Read the model definition and answer for the solid it produces. Units are mm, in the model's axes. A direction names the side the tool comes from. Give positions to 0.01 mm unless a question says otherwise; leave off trailing zeros. Write each loop counter-clockwise with the first axis right and the second up, starting at its lowest first coordinate (ties: lowest second). Pieces come first, ordered by that corner, then holes. Notation, with made-up numbers: (3, 87.25) -> (54, 87.25) arc R18 ccw to (54, 122.25) -> close; hole circle Ø6 at (12, 19.25). An arc over 180 degrees is marked (long way). Use a Markdown table: item, result.
from build123d import *

# Parameters (mm, degrees)
CHANFREIN2_SIZE  = 0.6
CHANFREIN2_SIZE2 = 0.218382141
CHANFREIN3_SIZE  = 0.3
CHANFREIN4_SIZE  = 0.2
CONG_1_R         = 0.4


with BuildPart() as part:
    # Esquisse1 → Base-Révolution (revolve)
    with BuildSketch(Plane.XY, mode=Mode.PRIVATE) as base_r_volution_sk:
        Polygon((-1, 6), (-1, 10), (0, 10), (0, 7), (8, 7), (8, 6), align=None)
    revolve(base_r_volution_sk.sketch.rotate(Axis((-5.312682662, 0, 0), (1, 0, 0)), 90), axis=Axis((-5.312682662, 0, 0), (1, 0, 0)))

    # Chanfrein2
    chanfrein2_edges = [part.edges().sort_by_distance(p)[0] for p in [
        (8, 0, -7),
    ]]
    chanfrein2_side = [part.faces().sort_by_distance(p)[0] for p in [
        (4, 0, -7),
    ]]
    chamfer(chanfrein2_edges, length=CHANFREIN2_SIZE, length2=CHANFREIN2_SIZE2, reference=chanfrein2_side[0])

    # Chanfrein3
    chanfrein3_edges = [part.edges().sort_by_distance(p)[0] for p in [
        (-1, 0, -6),
        (8, 0, -6),
    ]]
    chamfer(chanfrein3_edges, length=CHANFREIN3_SIZE)

    # Chanfrein4
    chanfrein4_edges = [part.edges().sort_by_distance(p)[0] for p in [
        (0, 0, -10),
        (-1, 0, -10),
    ]]
    chamfer(chanfrein4_edges, length=CHANFREIN4_SIZE)

    # Congé1
    cong_1_edges = [part.edges().sort_by_distance(p)[0] for p in [
        (0, 0, -7),
    ]]
    fillet(cong_1_edges, radius=CONG_1_R)


solid = part.part
Item 1: A cutting plane is placed at A-A (z = 0). Give the vertices of the cut face in (x, y), then the cut area to 3 significant figures.
Return value:
| item | result |
|---|---|
| outline | (-1, -9.8) -> (-0.8, -10) -> (-0.2, -10) -> (0, -9.8) -> (0, -7.4) arc R0.4 cw to (0.4, -7) -> (7.4, -7) -> (8, -6.78) -> (8, -6.3) -> (7.7, -6) -> (-0.7, -6) -> (-1, -6.3) -> close; (-1, 6.3) -> (-0.7, 6) -> (7.7, 6) -> (8, 6.3) -> (8, 6.78) -> (7.4, 7) -> (0.4, 7) arc R0.4 cw to (0, 7.4) -> (0, 9.8) -> (-0.2, 10) -> (-0.8, 10) -> (-1, 9.8) -> close |
| area | 23.7 mm^2 |
Item 2: Straight lines are drawn through the part: line 1 along Y through (x, z) = (1.25, 0); line 2 along Z through (x, y) = (5.75, 0.25); line 3 along X through (y, z) = (-6.75, 6.25). For each, find the intervals that lie inside material, in ascending order. Write a range as [from, to].
Return value:
| item | result |
|---|---|
| line 1 | [-7, -6], [6, 7] |
| line 2 | [-7, -5.99], [5.99, 7] |
| line 3 | [-1, 0] |
Item 3: A tool of negligible diameter and unlimited length cuts with its end or side. For faces 4 (the face through (3.95, 6.21, 3.23)), 5 (the face through (-1, 6.4, -2)), from which of +Z, -Z, +X, -X, +Y, -Y can it reach the whole face along a straight path? Write none if from no direction.
Return value:
| item | result |
|---|---|
| face 4 | +X |
| face 5 | +Z, -Z, -X, +Y, -Y |
Item 4: Each of these flat-tipped pins is pushed along its axis until it touches: P1, Ø5, axis at x = 7, z = -7.5, coming from the +Y side; P2, Ø4, axis at x = 6, z = 4, coming from the +Y side; P3, Ø5, axis at x = 1, y = -7, coming from the -Z side. Where does it stop, or does it pass through?
Return value:
| item | result |
|---|---|
| P1 | y = 4.9 |
| P2 | y = 6.71 |
| P3 | z = -8.77 |
Item 5: A cutting plane is placed at C-C (x = 3.75). Give the vertices of the cut face in (y, z).
Return value:
| item | result |
|---|---|
| outline | circle Ø14 at (0, 0); hole circle Ø12 at (0, 0) |
Item 6: For a pull along Z with two mould halves and no side action, classify faces 1 (the face through (3.441, -1.802, 5.723)), 2 (the face through (-0.5, -0.44, -9.99)), 3 (the face through (0, -7, -4)) as +Z half, -Z half, draft (parallel to the pull), parting line (faces both ways), or undercut.
Return value:
| item | result |
|---|---|
| face 1 | undercut |
| face 2 | parting line |
| face 3 | draft |
